Verification items for the finished model (mm, model axes). Face numbers are marked on the shaded views. A direction names the side the tool comes from. Give positions to 0.01 mm unless a question says otherwise; leave off trailing zeros. Loops run counter-clockwise (first coordinate to the right, second up) from the corner with the lowest first, then second, coordinate; pieces in that order, holes last. Notation, with made-up numbers: (-28.5, -26.75) - (-15.5, -26.75) arc R32 ccw to (-15.5, -0.75) - close; hole circle Ø9 at (61, 38). An arc over 180 degrees is marked (long way). One line per item, written item: value. Start each with the question number.
1. Sectioned sample at B-B (y = 0). Record the cut outline in (x, z).
2. Sectioned sample at C-C (x = 15.5). Record the cut outline in (y, z).
3. Scan lines: L1, parallel to Z at x = 3.75, y = 0.5; L2, parallel to X at y = -10, z = -17.5; L3, parallel to X at y = 3, z = -2. Record each from-to range of solid material in increasing order. Write a range as [from, to].
4. Sectioned sample at D-D (z = 5.5). Record the cut outline in (x, y), plus the area to 3 significant figures.
5. Access from +Z, -Z, +X, -X, +Y, -Y to the whole of each face (thin tool, end or side, straight path). Record for the marked faces 1 and 2.
6. Sectioned sample at A-A (z = 0). Record the cut outline in (x, y).
7. Gauge pin test, flat ends, axial feed: pin 1 (1.2 mm diameter, centred on x = 2, z = -7, fed in from +Y); pin 2 (6 mm diameter, centred on x = 8.5, z = -3.5, fed in from -Y); pin 3 (0.8 mm diameter, centred on x = 2, z = 8.5, fed in from +Y); pin 4 (5 mm diameter, centred on y = -8.5, z = 12, fed in from -X). Record the tip position at first contact, or that the pin passes through.
8. Mould release check, pull along Y, two halves, no side actions. Record for the marked faces 3, 4, 5 and 6: pulls with the +Y half, pulls with the -Y half, needs draft (parallel to the pull), parting line crosses it, or undercut.
from build123d import *

# Parameters (mm, degrees)
SKETCH1_R           = 22
BOSS_EXTRUDE1_DEPTH = 12
CUT_EXTRUDE2_DEPTH  = 5.5
SKETCH15_W          = 18
SKETCH15_H          = 24.118038922
CUT_EXTRUDE3_DEPTH  = 3
SKETCH16_R          = 4
BOSS_EXTRUDE2_DEPTH = 10
CUT_EXTRUDE4_START  = 22
SKETCH8_W           = 1.2
SKETCH8_H           = 10
CUT_EXTRUDE4_DEPTH  = 5
SKETCH17_W          = 4
SKETCH17_H          = 1.75
BOSS_EXTRUDE3_DEPTH = 1
SKETCH18_W          = 4.25
SKETCH18_H          = 1.737607108
BOSS_EXTRUDE4_DEPTH = 1
SKETCH22_R          = 1.5
CUT_EXTRUDE7_DEPTH  = 7


with BuildPart() as part:
    # Sketch1 → Boss-Extrude1 (new body)
    with BuildSketch(Plane(origin=(0, 0, 0), x_dir=(0, 0, -1), z_dir=(1, 0, 0))):
        Circle(SKETCH1_R)
    extrude(amount=BOSS_EXTRUDE1_DEPTH)

    # Sketch13 → Cut-Extrude2 (cut)
    with BuildSketch(Plane(origin=(0, 0, 0), x_dir=(0, 0, -1), z_dir=(1, 0, 0))):
        with BuildLine():
            Line((-2.670420152, -16.85816067), (-2.670420152, -16.530371213))
            Line((-2.670420152, -16.530371213), (-4.762392892, -10))
            Line((-4.762392892, -10), (-4.762392892, -6.943148259))
            Line((-4.762392892, -6.943148259), (-6.5, -6.943148259))
            Line((-6.5, -6.943148259), (-6.5, 19.556851741))
            Line((-6.5, 19.556851741), (6.5, 19.556851741))
            Line((6.5, 19.556851741), (6.5, -6.943148259))
            Line((6.5, -6.943148259), (4.762392892, -6.943148259))
            Line((4.762392892, -6.943148259), (4.762392892, -10))
            Line((4.762392892, -10), (2.670420152, -16.530371213))
            Line((2.670420152, -16.530371213), (2.670420152, -16.85816067))
            Line((2.670420152, -16.85816067), (2.670420152, -21.837327131))
            ThreePointArc((2.670420152, -21.837327131), (1.836835043, -21.92318492), (1.000584871, -21.977234355))
            Line((1.000584871, -21.977234355), (0, -25.25))
            Line((0, -25.25), (-1.000584871, -21.977234355))
            ThreePointArc((-1.000584871, -21.977234355), (-1.836835043, -21.92318492), (-2.670420152, -21.837327131))
            Line((-2.670420152, -21.837327131), (-2.670420152, -16.85816067))
        make_face()
    extrude(amount=CUT_EXTRUDE2_DEPTH, mode=Mode.SUBTRACT)

    # Sketch15 → Cut-Extrude3 (cut)
    with BuildSketch(Plane.ZY):
        with Locations((0, 5.115871202)):
            Rectangle(SKETCH15_W, SKETCH15_H)
    extrude(amount=-CUT_EXTRUDE3_DEPTH, mode=Mode.SUBTRACT)

    # Sketch16 → Boss-Extrude2 (add)
    with BuildSketch(Plane(origin=(12, 0, 0), x_dir=(0, 0, -1), z_dir=(1, 0, 0))):
        Circle(SKETCH16_R)
    extrude(amount=BOSS_EXTRUDE2_DEPTH)

    # Sketch8 → Cut-Extrude4 (cut)
    with BuildSketch(Plane(origin=(0, 0, 0), x_dir=(0, 0, -1), z_dir=(1, 0, 0)).offset(CUT_EXTRUDE4_START)):
        Rectangle(SKETCH8_W, SKETCH8_H)
    extrude(amount=-CUT_EXTRUDE4_DEPTH, mode=Mode.SUBTRACT)

    # Sketch17 → Boss-Extrude3 (add)
    with BuildSketch(Plane(origin=(0, -6.943148259, 0), x_dir=(1, 0, 0), z_dir=(0, 1, 0))):
        with Locations((2, 5.637392892)):
            Rectangle(SKETCH17_W, SKETCH17_H)
    extrude(amount=BOSS_EXTRUDE3_DEPTH)

    # Sketch18 → Boss-Extrude4 (add)
    with BuildSketch(Plane(origin=(0, -6.943148259, 0), x_dir=(1, 0, 0), z_dir=(0, 1, 0))):
        with Locations((2.125, -5.631196446)):
            Rectangle(SKETCH18_W, SKETCH18_H)
    extrude(amount=BOSS_EXTRUDE4_DEPTH)

    # Sketch22 → Cut-Extrude7 (cut)
    with BuildSketch(Plane(origin=(0, 0, 0), x_dir=(0, 0, -1), z_dir=(1, 0, 0))):
        with Locations((-14, 0)):
            Circle(SKETCH22_R)
        with Locations((14, 0)):
            Circle(SKETCH22_R)
    extrude(amount=CUT_EXTRUDE7_DEPTH, mode=Mode.SUBTRACT)


solid = part.part
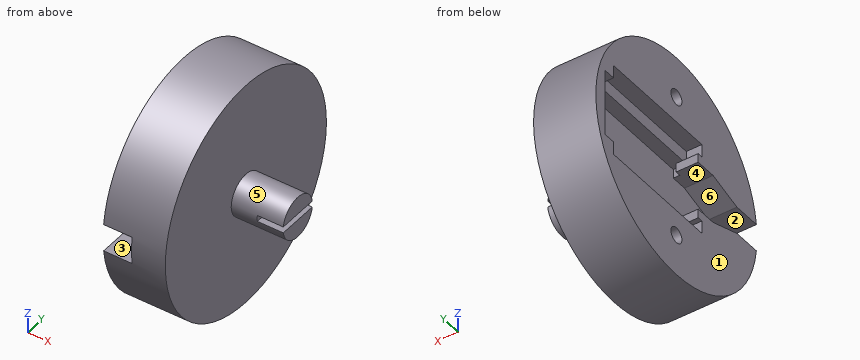
Results are:
1. outline: (0, -22) - (12, -22) - (12, -4) - (22, -4) - (22, -0.6) - (17, -0.6) - (17, 0.6) - (22, 0.6) - (22, 4) - (12, 4) - (12, 22) - (0, 22) - (0, 15.5) - (7, 15.5) - (7, 12.5) - (0, 12.5) - (0, 9) - (3, 9) - (3, 6.5) - (5.5, 6.5) - (5.5, -6.5) - (3, -6.5) - (3, -9) - (0, -9) - (0, -12.5) - (7, -12.5) - (7, -15.5) - (0, -15.5) - close
2. outline: circle Ø8 at (0, 0)
3. L1: z = [-21.99, -15.41], [-12.59, -6.5], [6.5, 12.59], [15.41, 21.99]
3. L2: x = [0, 12]
3. L3: x = [5.5, 22]
4. outline: (0, -21.3) - (12, -21.3) - (12, 21.3) - (0, 21.3) - (0, 19.56) - (5.5, 19.56) - (5.5, -6.94) - (4.25, -6.94) - (4.25, -5.94) - (0, -5.94) - close
4. area: 370 mm^2
5. face 1: +Z, -Z, -X, +Y, -Y
5. face 2: -X, -Y
6. outline: (0, 19.56) - (5.5, 19.56) - (5.5, -22) - (12, -22) - (12, -4) - (17, -4) - (17, 4) - (12, 4) - (12, 22) - (0, 22) - close
7. pin 1: stops at y = 21.05
7. pin 2: stops at y = -21.99
7. pin 3: stops at y = 20.45
7. pin 4: stops at x = 0
8. face 3: needs draft
8. face 4: undercut
8. face 5: parting line crosses it
8. face 6: undercut
